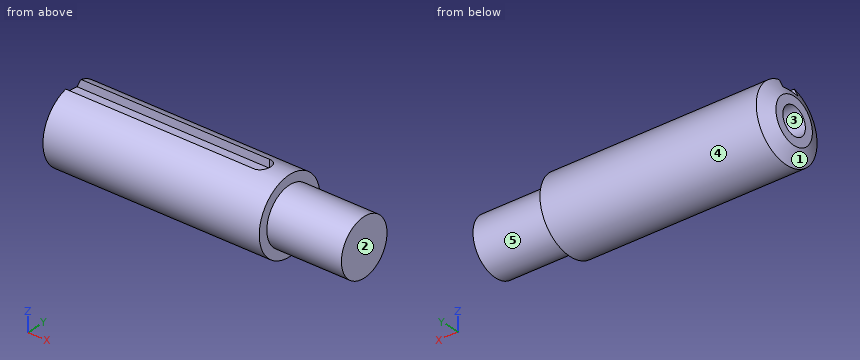
Autodesk Inventor part; units mm, degrees
ref_plane "YZ Plane" through (0, 0, 0) normal (1, 0, 0) x (0, 1, 0)
ref_plane "XZ Plane" through (0, 0, 0) normal (0, 1, 0) x (-1, 0, 0)
ref_plane "XY Plane" through (0, 0, 0) normal (0, 0, 1) x (1, 0, 0)
sketch "Sketch1" plane through (0, 0, 0) normal (1, 0, 0) x (0, 1, 0)
  circle A0 centre (0, 0) radius 6.35
  line L0 (0, 0) -> (0, 6.35) construction
  line L1 (-1.5875, 6.1484) -> (-1.5875, 4.7625)
  line L2 (-1.5875, 4.7625) -> (1.5875, 4.7625)
  line L3 (1.5875, 4.7625) -> (1.5875, 6.1484)
  point P0 (0, 4.7625)
  dimension "d0" = 12.7
  dimension "d2" = 1.5875
  dimension "d3" = 3.175
extrude "Extrusion1" add sketch "Sketch1" along normal blind 38.1
sketch "Sketch2" plane through (38.1, 0, 0) normal (1, 0, 0) x (0, 0, -1)
  circle A0 centre (0, 0) radius 6.35
  circle A1 centre (0, 0) radius 4.7625
  dimension "d6" = 9.525
extrude "Extrusion2" add sketch "Sketch2" along normal blind 12.7 contours A1
extrude "Extrusion3" cut sketch "Sketch1" along normal blind 34.925 contours L3 L2 L1 A0 picked at (0.1781, 5.2842)
fillet "Fillet1" radius 1.5875 2 edges at (34.925, 1.5875, 5.4554) (34.925, -1.5875, 5.4554)
chamfer "Chamfer1" distance 1.27 distance2 2.54 1 edges at (0, 0, -6.35) measured on face at (25.4, -3.3725, 5.3804)
sketch "Sketch3" plane through (0, 0, 0) normal (-1, 0, 0) x (0, 0, 1)
  circle A0 centre (0, 0) radius 3.81
  circle A1 centre (0, 0) radius 2.3495
  dimension "d16" = 4.699
extrude "Extrusion4" cut sketch "Sketch3" against normal blind 12.7 contours A1
thread "Thread1"
properties part number "Banebots 0.5x1.5 P60 Shaft" material "Steel, Carbon"
Check sheet for the modelled part. Datum: model origin and axes. Units: mm. Face numbers are marked on the shaded views. A direction names the side the tool comes from. Give positions to 0.01 mm unless a question says otherwise; leave off trailing zeros. Write each loop counter-clockwise with the first axis right and the second up, starting at its lowest first coordinate (ties: lowest second). Pieces come first, ordered by that corner, then holes. Notation, with made-up numbers: (87, -39) -> (129, -39) arc R26 ccw to (129, -10) -> close; hole circle Ø1 at (-38.75, 78.25). An arc over 180 degrees is marked (long way). Use one line per item in the form item = value. Start each with the question number.
1. Section check C-C (x = 5). Record the cut outline in (y, z), and give its area (3 significant figures).
2. Go/stop test with flat-tipped pins: P1, Ø2.5, axis at x = 20.5, y = 0, coming from the +Z side; P2, Ø4, axis at y = 0, z = 0, coming from the -X side; P3, Ø1, axis at x = 7, y = -3, coming from the +Z side. Record where each tip stops, or that it passes through.
3. Thickness scan on line 1 along Y through (x, z) = (3.5, 0); line 2 along Y through (x, z) = (26, -0.25); line 3 along X through (y, z) = (-2, 0.75). Record the ranges inside material, lowest first. Write a range as from..to.
4. Section check D-D (x = 23). Record the cut outline in (y, z), and give its area (3 significant figures).
5. Access from +Z, -Z, +X, -X, +Y, -Y to the whole of each face (thin tool, end or side, straight path). Record for the marked faces 4 and 5.
6. Mould release check, pull along X, two halves, no side actions. Record for the marked faces 1, 2 and 3: pulls with the +X half, pulls with the -X half, needs draft (parallel to the pull), parting line crosses it, or undercut.
7. Section check A-A (z = 0). Record the cut outline in (x, y), and give its area (3 significant figures).
Conclusion:
q1.outline = (-1.59, 4.76) -> (-1.59, 6.15) arc R6.35 ccw (long way) to (1.59, 6.15) -> (1.59, 4.76) -> close; hole circle Ø4.7 at (0, 0)
q1.area = 105 mm²
q2.P1 = 4.76
q2.P2 = 12.7
q2.P3 = 5.84
q3.line_1 = -6.35..-2.35, 2.35..6.35
q3.line_2 = -6.35..6.35
q3.line_3 = 12.7..50.8
q4.outline = (-1.59, 4.76) -> (-1.59, 6.15) arc R6.35 ccw (long way) to (1.59, 6.15) -> (1.59, 4.76) -> close
q4.area = 122 mm²
q5.face_4 = +X, -X
q5.face_5 = +X
q6.face_1 = pulls with the -X half
q6.face_2 = pulls with the +X half
q6.face_3 = needs draft
q7.outline = (0, -3.81) -> (1.27, -6.35) -> (38.1, -6.35) -> (38.1, -4.76) -> (50.8, -4.76) -> (50.8, 4.76) -> (38.1, 4.76) -> (38.1, 6.35) -> (1.27, 6.35) -> (0, 3.81) -> (0, 2.35) -> (12.7, 2.35) -> (12.7, -2.35) -> (0, -2.35) -> close
q7.area = 542 mm²
